Design review of the part built by this model. Coordinates are the model's own, in mm. A direction names the side the tool comes from. Coordinates: 2 decimals unless noted, no trailing zeros. Loops run counter-clockwise (first coordinate to the right, second up) from the corner with the lowest first, then second, coordinate; pieces in that order, holes last. Notation, with made-up numbers: (77, 33.25) - (133, 33.25) arc R17 ccw to (133, 66.25) - close; hole circle Ø9 at (70, 51.25). An arc over 180 degrees is marked (long way). Answer in a Markdown table with one row per item. Add a question column.
(1) The part is to be moulded in two halves that separate along Y. For faces 1 (the face through (-3, 12.5, 3)), 2 (the face through (142.5, -3, 2)), 3 (the face through (-3, 62.5, 3)), say which applies: released by +Y, released by -Y, zero draft, split by the parting line, or undercut.
(2) Clearance check with flat-ended pins moving along their axes: pin 1 (1.5 mm diameter, centred on x = -3, z = 2, fed in from +Y); pin 2 (1.5 mm diameter, centred on x = 85.5, z = 2, fed in from -Y); pin 3 (1.5 mm diameter, centred on y = 44, z = 3, fed in from -X). State where each tip first meets the part, or that it passes through.
(3) For faces 4 (the face through (0, 6, 2)), 5 (the face through (149, 0, 2)), 6 (the face through (-3, 37.5, 3)), list the 3-axis set-ups (+Z, -Z, +X, -X, +Y, -Y) from which the entire face can be reached by the end or side of a thin tool; tool diameter is ignored.
(4) To check wall thickness, follow L1, parallel to X at y = 46.5, z = 1.55; L2, parallel to Y at x = 14.5, z = 1.4. State the ranges of each line that lie inside material, in increasing order. Write a range as [from, to].
(5) We need section A-A, the plane z = 3.3. Write out the cut boundary in (x, y), plus the area to 3 significant figures.
(6) We need section B-B, the plane y = 57. Write out the cut boundary in (x, z), plus the area to 3 significant figures.
(7) We need section C-C, the plane x = 87. Write out the cut boundary in (y, z), plus the area to 3 significant figures.
from build123d import *

# Parameters (mm, degrees)
CROQUIS1_W              = 5
CROQUIS1_H              = 25
SALIENTE_EXTRUIR1_DEPTH = 5
CROQUIS3_W              = 5
CROQUIS3_H              = 25
SALIENTE_EXTRUIR2_DEPTH = 5


with BuildPart() as part:
    # Croquis1 → Saliente-Extruir1 (new body)
    with BuildSketch(Plane.XY):
        Polygon((0, 12.5), (0, 0), (17.5, 0), (17.5, -5), (62.5, -5), (62.5, 0), (97.5, 0), (97.5, -5), (142.5, -5), (142.5, 0), (155, 0), (155, 100), (0, 100), (0, 87.5), (5, 87.5), (5, 62.5), (0, 62.5), (0, 37.5), (5, 37.5), (5, 12.5), align=None)
        with Locations((2.5, 25)):
            Rectangle(CROQUIS1_W, CROQUIS1_H)
        with Locations((2.5, 75)):
            Rectangle(CROQUIS1_W, CROQUIS1_H)
    extrude(amount=SALIENTE_EXTRUIR1_DEPTH)

    # Croquis3 → Saliente-Extruir2 (add)
    with BuildSketch(Plane.XY.offset(5)):
        with Locations((-2.5, 25)):
            Rectangle(CROQUIS3_W, CROQUIS3_H)
        with Locations((-2.5, 75)):
            Rectangle(CROQUIS3_W, CROQUIS3_H)
    extrude(amount=-SALIENTE_EXTRUIR2_DEPTH)


solid = part.part
Responses:
| question | item | result |
|---|---|---|
| 1 | face 1 | released by -Y |
| 1 | face 2 | zero draft |
| 1 | face 3 | undercut |
| 2 | pin 1 | stops at y = 87.5 |
| 2 | pin 2 | stops at y = 0 |
| 2 | pin 3 | stops at x = 0 |
| 3 | face 4 | +Z, -Z, -X, -Y |
| 3 | face 5 | +Z, -Z, +X, -Y |
| 3 | face 6 | +Z, -Z, -X |
| 4 | L1 | x = [0, 155] |
| 4 | L2 | y = [0, 100] |
| 5 | outline | (-5, 12.5) - (0, 12.5) - (0, 0) - (17.5, 0) - (17.5, -5) - (62.5, -5) - (62.5, 0) - (97.5, 0) - (97.5, -5) - (142.5, -5) - (142.5, 0) - (155, 0) - (155, 100) - (0, 100) - (0, 87.5) - (-5, 87.5) - (-5, 62.5) - (0, 62.5) - (0, 37.5) - (-5, 37.5) - close |
| 5 | area | 16,200 mm2 |
| 6 | outline | (0, 0) - (155, 0) - (155, 5) - (0, 5) - close |
| 6 | area | 775 mm2 |
| 7 | outline | (0, 0) - (100, 0) - (100, 5) - (0, 5) - close |
| 7 | area | 500 mm2 |
